from build123d import *

# Parameters (mm, degrees)
SKETCH1_R                = 13.365
BOSS_EXTRUDE1_DEPTH      = 10
SKETCH2_R                = 15
BOSS_EXTRUDE2_DEPTH      = 2
BOSS_EXTRUDE3_START      = -2
SKETCH3_R                = 15
BOSS_EXTRUDE3_DEPTH      = 2
BOSS_EXTRUDE4_DEPTH      = 30
BOSS_EXTRUDE4_DEPTH_BACK = 65
SKETCH4_R                = 6.365
SKETCH5_R                = 8.5
BOSS_EXTRUDE5_DEPTH      = 10
BOSS_EXTRUDE6_START      = -10
SKETCH6_R                = 8.5
BOSS_EXTRUDE6_DEPTH      = 10
SKETCH7_R                = 8.5
BOSS_EXTRUDE7_DEPTH      = 63


with BuildPart() as part:
    # Sketch1 → Boss-Extrude1 (new body)
    with BuildSketch(Plane(origin=(0, 0, 0), x_dir=(1, 0, 0), z_dir=(0, 1, 0))):
        with Locations(Location((0, 0, 0), (0, 0, 270))):
            Circle(SKETCH1_R)
    extrude(amount=BOSS_EXTRUDE1_DEPTH)

    # Sketch2 → Boss-Extrude2 (add)
    with BuildSketch(Plane(origin=(0, 10, 0), x_dir=(1, 0, 0), z_dir=(0, 1, 0))):
        with Locations(Location((0, 0, 0), (0, 0, 270))):
            Circle(SKETCH2_R)
    extrude(amount=-BOSS_EXTRUDE2_DEPTH)

    # Sketch3 → Boss-Extrude3 (add)
    with BuildSketch(Plane.XZ.offset(BOSS_EXTRUDE3_START)):
        with Locations(Location((0, 0, 0), (0, 0, 90))):
            Circle(SKETCH3_R)
    extrude(amount=BOSS_EXTRUDE3_DEPTH)

    # Sketch4 → Boss-Extrude4 (add, two sides: drawn at the far end of the back side and taken through both)
    with BuildSketch(Plane.XZ.offset(-BOSS_EXTRUDE4_DEPTH_BACK)):
        with Locations(Location((0, 0, 0), (0, 0, 270))):
            Circle(SKETCH4_R)
    extrude(amount=BOSS_EXTRUDE4_DEPTH + BOSS_EXTRUDE4_DEPTH_BACK)

    # Sketch5 → Boss-Extrude5 (add)
    with BuildSketch(Plane.XZ.offset(30)):
        with Locations(Location((0, 0, 0), (0, 0, 270))):
            Circle(SKETCH5_R)
    extrude(amount=-BOSS_EXTRUDE5_DEPTH)

    # Sketch6 → Boss-Extrude6 (add)
    with BuildSketch(Plane(origin=(0, 65, 0), x_dir=(1, 0, 0), z_dir=(0, 1, 0)).offset(BOSS_EXTRUDE6_START)):
        with Locations(Location((0, 0, 0), (0, 0, 90))):
            Circle(SKETCH6_R)
    extrude(amount=BOSS_EXTRUDE6_DEPTH)

    # Sketch7 → Boss-Extrude7 (add)
    with BuildSketch(Plane(origin=(0, -14, 0), x_dir=(1, 0, 0), z_dir=(0, 1, 0))):
        with Locations(Location((0, 0, 0), (0, 0, 270))):
            Circle(SKETCH7_R)
    extrude(amount=BOSS_EXTRUDE7_DEPTH)


solid = part.part
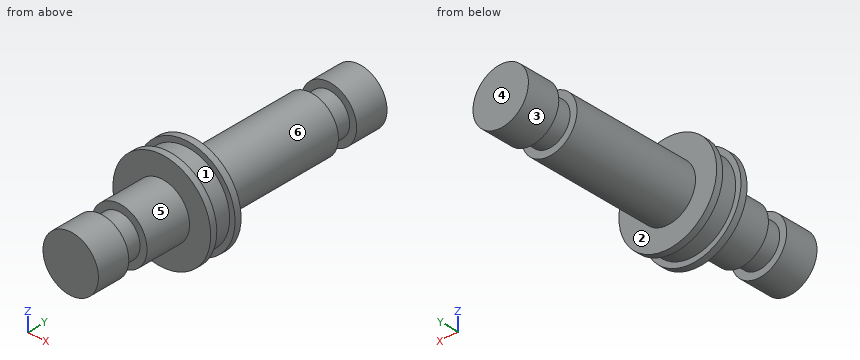
Geometry check sheet. Reference: the model listing, model coordinates, mm. Face numbers are marked on the shaded views. A direction names the side the tool comes from. Round coordinates to 2 decimals unless told otherwise and drop trailing zeros. Loops run counter-clockwise (first coordinate to the right, second up) from the corner with the lowest first, then second, coordinate; pieces in that order, holes last.
Item 1: Cross-section at A-A on x = 7.25. Record the boundary of the cut face in (y, z), then the cut area to 3 significant figures.
Item 2: Cross-section at C-C on y = 54. Record the boundary of the cut face in (x, z) (3 decimals).
Item 3: Thickness scan on line 1 (Y direction, x = 3, z = -6.5); line 2 (X direction, y = 22, z = 0); line 3 (Y direction, x = 2, z = -13). Record the ranges inside material, lowest first.
Item 4: Gauge pin test, flat ends, axial feed: pin 1 (9 mm diameter, centred on x = 6.5, z = -6.5, fed in from -Y); pin 2 (3 mm diameter, centred on x = -1, y = -3.5, fed in from +Z); pin 3 (1.5 mm diameter, centred on x = -5.5, z = -11, fed in from -Y); pin 4 (3 mm diameter, centred on x = 5.5, y = -0.5, fed in from -Z). Record the tip position at first contact, or that the pin passes through.
Item 5: Cross-section at B-B on z = 10.75. Record the boundary of the cut face in (x, y), then the cut area to 3 significant figures.
Item 6: Cross-section at D-D on x = -11.5. Record the boundary of the cut face in (y, z), then the cut area to 3 significant figures.
Item 7: Mould release check, pull along Y, two halves, no side actions. Record for the marked faces 1, 2 and 3: pulls with the +Y half, pulls with the -Y half, needs draft (parallel to the pull), parting line crosses it, or undercut.
Item 8: Access from +Z, -Z, +X, -X, +Y, -Y to the whole of each face (thin tool, end or side, straight path). Record for the marked faces 4, 5 and 6.
Answer sheet:
1. outline: (-30, -4.44) - (-20, -4.44) - (-20, 4.44) - (-30, 4.44) - close; (-14, -4.44) - (0, -4.44) - (0, -13.13) - (2, -13.13) - (2, -11.23) - (8, -11.23) - (8, -13.13) - (10, -13.13) - (10, -4.44) - (49, -4.44) - (49, 4.44) - (10, 4.44) - (10, 13.13) - (8, 13.13) - (8, 11.23) - (2, 11.23) - (2, 13.13) - (0, 13.13) - (0, 4.44) - (-14, 4.44) - close; (55, -4.44) - (65, -4.44) - (65, 4.44) - (55, 4.44) - close
1. area: 888 mm2
2. outline: circle Ø12.73 at (0, 0)
3. line 1: y = -30 to -20, -14 to 49, 55 to 65
3. line 2: x = -8.5 to 8.5
3. line 3: y = 0 to 10
4. pin 1: stops at y = -30
4. pin 2: stops at z = 8.5
4. pin 3: stops at y = 0
4. pin 4: stops at z = -14.43
5. outline: (-10.46, 0) - (10.46, 0) - (10.46, 2) - (7.94, 2) - (7.94, 8) - (10.46, 8) - (10.46, 10) - (-10.46, 10) - (-10.46, 8) - (-7.94, 8) - (-7.94, 2) - (-10.46, 2) - close
5. area: 179 mm2
6. outline: (0, -9.63) - (2, -9.63) - (2, -6.81) - (8, -6.81) - (8, -9.63) - (10, -9.63) - (10, 9.63) - (8, 9.63) - (8, 6.81) - (2, 6.81) - (2, 9.63) - (0, 9.63) - close
6. area: 159 mm2
7. face 1: undercut
7. face 2: pulls with the +Y half
7. face 3: needs draft
8. face 4: +Z, -Z, +X, -X, +Y
8. face 5: -Y
8. face 6: +Y
